Read the model definition and answer for the solid it produces. Units are mm, in the model's axes. Face numbers are marked on the shaded views. Coordinates: 2 decimals unless noted, no trailing zeros. Write each loop counter-clockwise with the first axis right and the second up, starting at its lowest first coordinate (ties: lowest second). Pieces come first, ordered by that corner, then holes. Notation, with made-up numbers: (-30.75, 6.5) -> (-22.75, 6.5) arc R25 ccw to (-22.75, 19.5) -> close; hole circle Ø5 at (-11.75, 45.25). An arc over 180 degrees is marked (long way). One line per item, written item: value. Start each with the question number.
from build123d import *

# Parameters (mm, degrees)
SKETCH1_W           = 210
SKETCH1_H           = 210
MAINEXTRUDE_DEPTH   = 4
SKETCH1_6_R         = 1.5
SCREWHOLES_DEPTH    = 4
ROUNDEDCORNERS_R    = 10
TRENCH_DEPTH        = 12
TRENCH_WALLS_DEPTH  = 10
TRENCH_BOTTOM_DEPTH = 2


with BuildPart() as part:
    # Sketch1 → MainExtrude (new body)
    with BuildSketch(Plane(origin=(0, 0, 0), x_dir=(1, 0, 0), z_dir=(0, 1, 0))):
        Rectangle(SKETCH1_W, SKETCH1_H)
    extrude(amount=MAINEXTRUDE_DEPTH)

    # Sketch1<6> → ScrewHoles (cut)
    with BuildSketch(Plane(origin=(0, 0, 0), x_dir=(1, 0, 0), z_dir=(0, 1, 0))):
        with Locations((-99.833273811, 99.833273811)):
            Circle(SKETCH1_6_R)
        with Locations((-99.833273811, -99.833273811)):
            Circle(SKETCH1_6_R)
        with Locations((99.833273811, -99.833273811)):
            Circle(SKETCH1_6_R)
        with Locations((99.833273811, 99.833273811)):
            Circle(SKETCH1_6_R)
    extrude(amount=SCREWHOLES_DEPTH, mode=Mode.SUBTRACT)

    # RoundedCorners
    roundedcorners_edges = [part.edges().sort_by_distance(p)[0] for p in [
        (-105, 2, -105),
        (-105, 2, 105),
        (105, 2, 105),
        (105, 2, -105),
    ]]
    fillet(roundedcorners_edges, radius=ROUNDEDCORNERS_R)

    # Sketch3 → Trench (cut)
    with BuildSketch(Plane(origin=(0, 0, 0), x_dir=(1, 0, 0), z_dir=(0, 1, 0))):
        Polygon((-57, 93), (-57, 33), (-93, 33), (-93, 23), (57, 23), (57, -43), (-83, -43), (-83, -13), (37, -13), (37, -3), (-93, -3), (-93, -53), (-27, -53), (-27, -93), (93, -93), (93, 87), (-27, 87), (-27, 77), (83, 77), (83, -83), (-17, -83), (-17, -53), (67, -53), (67, 33), (-47, 33), (-47, 93), align=None)
    extrude(amount=TRENCH_DEPTH, mode=Mode.SUBTRACT)

    # Sketch7 → Trench Walls (add)
    with BuildSketch(Plane.XZ):
        Polygon((-59, -95), (-45, -95), (-45, -35), (69, -35), (69, 55), (-15, 55), (-15, 81), (81, 81), (81, -75), (-29, -75), (-29, -89), (95, -89), (95, 95), (-29, 95), (-29, 55), (-95, 55), (-95, 1), (39, 1), (39, 15), (-81, 15), (-81, 41), (55, 41), (55, -21), (-95, -21), (-95, -35), (-59, -35), align=None)
        Polygon((-57, -93), (-47, -93), (-47, -33), (67, -33), (67, 53), (-17, 53), (-17, 83), (83, 83), (83, -77), (-27, -77), (-27, -87), (93, -87), (93, 93), (-27, 93), (-27, 53), (-93, 53), (-93, 3), (37, 3), (37, 13), (-83, 13), (-83, 43), (57, 43), (57, -23), (-93, -23), (-93, -33), (-57, -33), align=None, mode=Mode.SUBTRACT)
    extrude(amount=TRENCH_WALLS_DEPTH)

    # Sketch8 → Trench Bottom (add)
    with BuildSketch(Plane.XZ.offset(10)):
        Polygon((-59, -35), (-59, -95), (-45, -95), (-45, -35), (69, -35), (69, 55), (-15, 55), (-15, 81), (81, 81), (81, -75), (-29, -75), (-29, -89), (95, -89), (95, 95), (-29, 95), (-29, 55), (-95, 55), (-95, 1), (39, 1), (39, 15), (-81, 15), (-81, 41), (55, 41), (55, -21), (-95, -21), (-95, -35), align=None)
    extrude(amount=TRENCH_BOTTOM_DEPTH)


solid = part.part
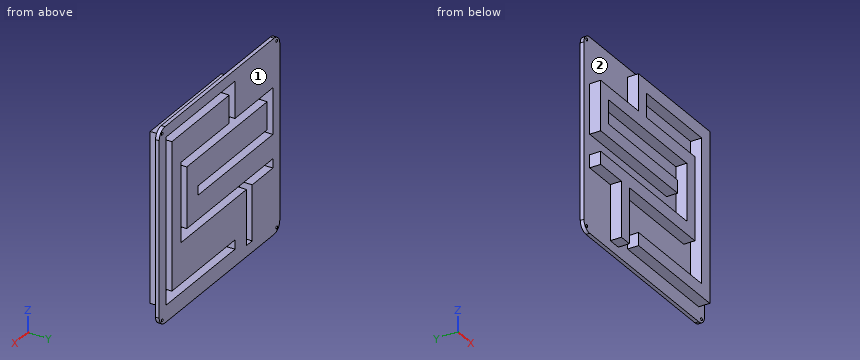
1. Find the intervals of material crossed by probe 1 along X at (y, z) = (-4, 37.5); probe 2 along X at (y, z) = (-9.75, -18); probe 3 along X at (y, z) = (-9.25, -77.5), in increasing order. Write a range as from..to.
2. Given pin 1 (5 mm diameter, centred on y = -7.5, z = -53.5, fed in from -X); pin 2 (4 mm diameter, centred on y = -5.5, z = 68.5, fed in from -X); pin 3 (1.5 mm diameter, centred on y = -9.5, z = 43, fed in from +X), each flat-ended and moving along its own axis, determine where each tip first touches the part or whether it passes through.
3. A cutting plane is placed at C-C on z = -64.5. Give the vertices of the cut face in (x, y).
4. A cutting plane is placed at A-A on z = 30. Give the vertices of the cut face in (x, y).
5. A cutting plane is placed at B-B on x = -87.5. Give the vertices of the cut face in (y, z).
6. A cutting plane is placed at D-D on x = -38.5. Give the vertices of the cut face in (y, z), then the cut area to 3 significant figures.
7. For a pull along X with two mould halves and no side action, classify the marked faces 1 and 2 as +X half, -X half, draft (parallel to the pull), parting line (faces both ways), or undercut.
Derived:
1. probe 1: x = -95..-93, -83..-81, 55..57, 67..69, 81..83, 93..95
1. probe 2: x = 55..57, 67..69, 81..83, 93..95
1. probe 3: x = -59..-57, -47..-45, -29..-27, 93..95
2. pin 1: stops at x = -59
2. pin 2: stops at x = -29
2. pin 3: stops at x = 95
3. outline: (-105, 0) -> (-59, 0) -> (-59, -12) -> (-45, -12) -> (-45, 0) -> (81, 0) -> (81, -12) -> (95, -12) -> (95, 0) -> (105, 0) -> (105, 4) -> (93, 4) -> (93, -10) -> (83, -10) -> (83, 4) -> (-47, 4) -> (-47, -10) -> (-57, -10) -> (-57, 4) -> (-105, 4) -> close
4. outline: (-105, 0) -> (-95, 0) -> (-95, -12) -> (-81, -12) -> (-81, 0) -> (55, 0) -> (55, -12) -> (69, -12) -> (69, 0) -> (81, 0) -> (81, -12) -> (95, -12) -> (95, 0) -> (105, 0) -> (105, 4) -> (93, 4) -> (93, -10) -> (83, -10) -> (83, 4) -> (67, 4) -> (67, -10) -> (57, -10) -> (57, 4) -> (-83, 4) -> (-83, -10) -> (-93, -10) -> (-93, 4) -> (-105, 4) -> close
5. outline: (-12, -35) -> (0, -35) -> (0, -105) -> (4, -105) -> (4, -33) -> (-10, -33) -> (-10, -23) -> (4, -23) -> (4, 3) -> (-10, 3) -> (-10, 53) -> (4, 53) -> (4, 105) -> (0, 105) -> (0, 55) -> (-12, 55) -> (-12, 1) -> (0, 1) -> (0, -21) -> (-12, -21) -> close
6. outline: (-12, -35) -> (0, -35) -> (0, -105) -> (4, -105) -> (4, -33) -> (-10, -33) -> (-10, -23) -> (4, -23) -> (4, 3) -> (-10, 3) -> (-10, 13) -> (4, 13) -> (4, 43) -> (-10, 43) -> (-10, 53) -> (4, 53) -> (4, 105) -> (0, 105) -> (0, 55) -> (-12, 55) -> (-12, 41) -> (0, 41) -> (0, 15) -> (-12, 15) -> (-12, 1) -> (0, 1) -> (0, -21) -> (-12, -21) -> close
6. area: 924 mm2
7. face 1: draft
7. face 2: undercut
